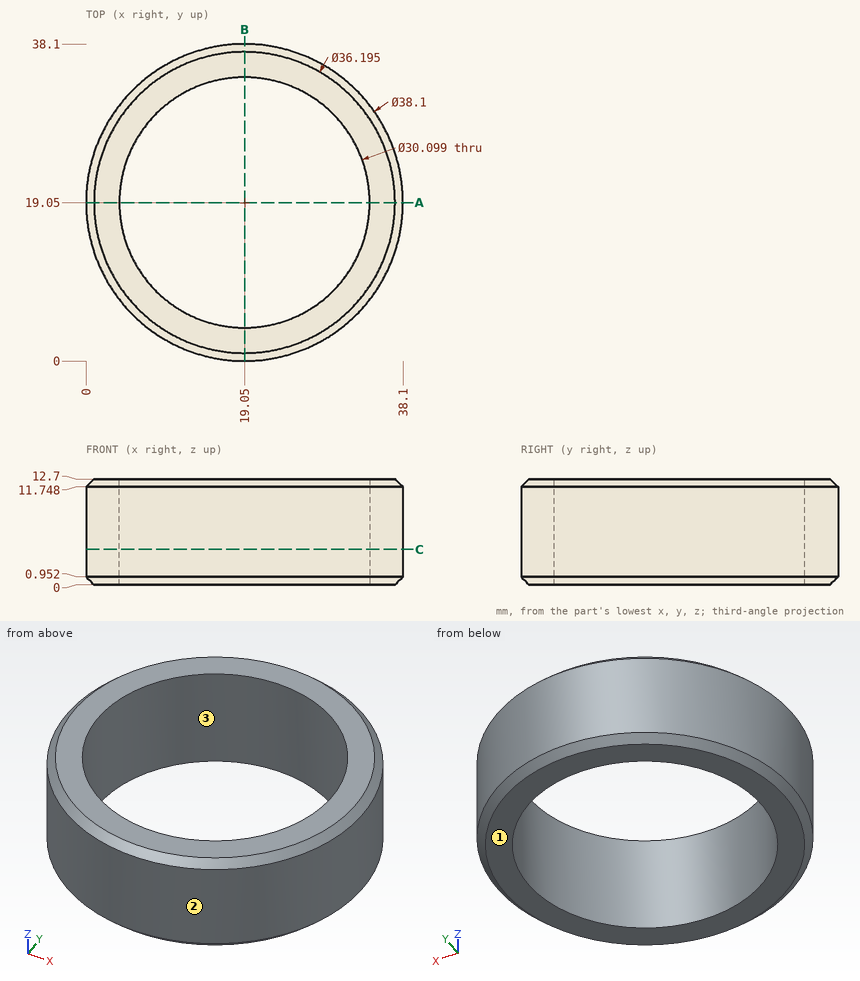
Can you work these out from the drawing? Everything is in mm from the part's minimum corner. Coordinates: 2 decimals unless noted, no trailing zeros. Order: outer loops, then holes, each group sorted by start corner. A loop starts at its lowest first (then second) coordinate and runs counter-clockwise, first axis right, second up. Notation, with made-up numbers: (-37.75, 21.25) -> (9.25, 21.25) arc R3 ccw to (9.25, 25.25) -> close; hole circle Ø10 at (82, -15.75). An arc over 180 degrees is marked (long way). Return JSON: item names as keys, results as strings.
1) If we section it at A-A on y = 19.05: List the corners of the cut face in (x, z) for me.
Conclusion:
{"outline": "(0, 0.95) -> (0.95, 0) -> (4, 0) -> (4, 12.7) -> (0.95, 12.7) -> (0, 11.75) -> close; (34.1, 0) -> (37.15, 0) -> (38.1, 0.95) -> (38.1, 11.75) -> (37.15, 12.7) -> (34.1, 12.7) -> close"}
2) If we section it at C-C on z = 4.25: List the corners of the cut face in (x, y) for me.
Conclusion:
{"outline": "circle Ø38.1 at (19.05, 19.05); hole circle Ø30.1 at (19.05, 19.05)"}
3) Thinking about a two-plate mould opening in X: for the marked faces 1, 2 and 3, which applies, +X half, -X half, draft (parallel to the pull), parting line (faces both ways), or undercut?
Conclusion:
{"face 1": "draft", "face 2": "parting line", "face 3": "undercut"}
4) If I drill on probe 1 along Y at (x, z) = (19.05, 7.75); probe 2 along Y at (x, z) = (31, 4) (1 decimal); probe 3 along X at (y, z) = (28.5, 11.75) (1 decimal), over which ranges is the centre line in solid material (lowest first)?
Conclusion:
{"probe 1": "y = 0 to 4, 34.1 to 38.1", "probe 2": "y = 4.2 to 9.9, 28.2 to 33.9", "probe 3": "x = 2.5 to 7.3, 30.8 to 35.6"}
5) I'm going to push flat-ended pins straight in: P1, Ø1.5, axis at y = 7.5, z = 5.5, coming from the +X side; P2, Ø4, axis at y = 28, z = 2, coming from the +X side; P3, Ø5, axis at y = 33, z = 4, coming from the +X side (1 decimal); P4, Ø1.5, axis at x = 27.5, y = 9.5, coming from the +Z side. Where does each tip first touch, or does it pass through?
Conclusion:
{"P1": "stops at x = 34.74", "P2": "stops at x = 36.79", "P3": "stops at x = 34.3", "P4": "passes through"}
